Input: part model. Units: mm. Frame: model coordinates. A direction names the side the tool comes from. Coordinates: 2 decimals unless noted, no trailing zeros. Order: outer loops, then holes, each group sorted by start corner. A loop starts at its lowest first (then second) coordinate and runs counter-clockwise, first axis right, second up. Notation, with made-up numbers: M 19,-29.5 L 24,-29.5 A28 cw 24,5.5 Z; hole C 77.25,56.5 d10. An arc over 180 degrees is marked long. One line per item, written item: value.
```python
from build123d import *

# Parameters (mm, degrees)
F0_R     = 12.95
F0_R_2   = 10.95
F1_DEPTH = 3


with BuildPart() as f1:
    # F0 (on Top) → F1 (new body)
    with BuildSketch(Plane.XY):
        with BuildLine():
            Line((30, 15), (-30, 15))
            ThreePointArc((-30, 15), (-55, 0), (-30, -15))
            Line((-30, -15), (0, -15))
            Line((0, -15), (30, -15))
            ThreePointArc((30, -15), (55, 0), (30, 15))
        make_face()
        with Locations((-38, 0)):
            Circle(F0_R, mode=Mode.SUBTRACT)
        Circle(F0_R_2, mode=Mode.SUBTRACT)
        with Locations((38, 0)):
            Circle(F0_R, mode=Mode.SUBTRACT)
    extrude(amount=F1_DEPTH)


solid = f1.part
```
(1) First-contact query: pin 1 (1.5 mm diameter, centred on x = -10.5, z = 2, fed in from +Y); pin 2 (1.5 mm diameter, centred on x = -6.5, z = 2.5, fed in from -Y). Flat tips, straight axial feed; report the tip coordinate or a pass-through.
Data:
pin 1: stops at y = 15
pin 2: stops at y = -15
(2) Cut plane C-C on z = 2.55. Output: boundary loops of the cut face in (x, y).
Data:
outline: M -30,-15 L 30,-15 A17 ccw long 30,15 L -30,15 A17 ccw long Z; hole C -38,0 d25.9; hole C 0,0 d21.9; hole C 38,0 d25.9
(3) Cut plane B-B on y = 0. Output: boundary loops of the cut face in (x, z).
Data:
outline: M -55,0 L -50.95,0 L -50.95,3 L -55,3 Z; M -25.05,0 L -10.95,0 L -10.95,3 L -25.05,3 Z; M 10.95,0 L 25.05,0 L 25.05,3 L 10.95,3 Z; M 50.95,0 L 55,0 L 55,3 L 50.95,3 Z
(4) Ray query, line 1 (Y direction, x = 38, z = 1.4); line 2 (Y direction, x = 0, z = 1.35); line 3 (X direction, y = -4, z = 2.75). Return the intervals inside material, ascending. Write a range as from..to.
Data:
line 1: y = -17..-12.95, 12.95..17
line 2: y = -15..-10.95, 10.95..15
line 3: x = -54.52..-50.32, -25.68..-10.19, 10.19..25.68, 50.32..54.52
(5) Access query for faces 5 (the flat face through (0, -15, 1)), 6 (the cylindrical face through (55, 0, 1)), 7 (the flat face through (0, 15, 1)). Directions: +Z, -Z, +X, -X, +Y, -Y. A direction counts if a zero-diameter tool reaches every point of the face in a straight line with its end or side. Return the directions, or none.
Data:
face 5: +Z, -Z, -Y
face 6: +Z, -Z
face 7: +Z, -Z, +Y
(6) Cut plane D-D on y = -4.5. Output: boundary loops of the cut face in (x, z).
Data:
outline: M -54.39,0 L -50.14,0 L -50.14,3 L -54.39,3 Z; M -25.86,0 L -9.98,0 L -9.98,3 L -25.86,3 Z; M 9.98,0 L 25.86,0 L 25.86,3 L 9.98,3 Z; M 50.14,0 L 54.39,0 L 54.39,3 L 50.14,3 Z
(7) Draft query along Y for faces 1 (the flat face through (-0.8, -11.1, 3)), 2 (the cylindrical face through (-8.69, -6.66, 1.48)), 3 (the cylindrical face through (-50.937, 0.569, 1.479)), 4 (the cylindrical face through (-55, 0, 1)). Return one class per face: released by +Y, released by -Y, zero draft, split by the parting line, or undercut.
Data:
face 1: zero draft
face 2: undercut
face 3: undercut
face 4: split by the parting line
(8) Cut plane A-A on x = -38. Output: boundary loops of the cut face in (y, z), plus the area to 3 significant figures.
Data:
outline: M -17,0 L -12.95,0 L -12.95,3 L -17,3 Z; M 12.95,0 L 17,0 L 17,3 L 12.95,3 Z
area: 24.3 mm2
